Geometry check sheet. Reference: drawing and pictorial views, mm from the part's lowest x, y, z. Coordinates: 2 decimals unless noted, no trailing zeros. Loops run counter-clockwise (first coordinate to the right, second up) from the corner with the lowest first, then second, coordinate; pieces in that order, holes last.
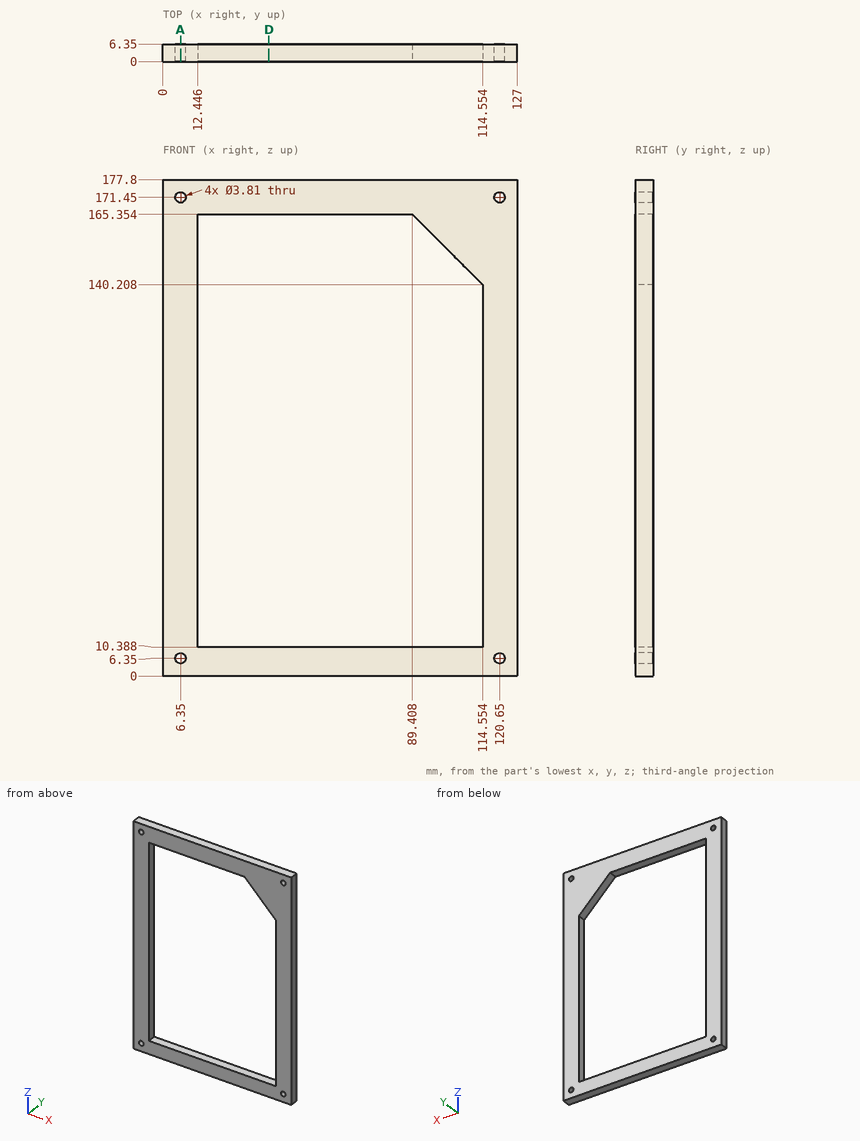
1) Section check D-D on x = 38. Record the cut outline in (y, z), and give its area (3 significant figures).
Data:
outline: (0, 0) - (6.35, 0) - (6.35, 10.39) - (0, 10.39) - close; (0, 165.35) - (6.35, 165.35) - (6.35, 177.8) - (0, 177.8) - close
area: 145 mm2
2) Material ranges on probe 1 along X at (y, z) = (4.5, 6.35) (1 decimal); probe 2 along Z at (x, y) = (64, 3.75); probe 3 along X at (y, z) = (3.5, 47), recorded low to high.
Data:
probe 1: x = 0 to 4.4, 8.3 to 118.7, 122.6 to 127
probe 2: z = 0 to 10.39, 165.35 to 177.8
probe 3: x = 0 to 12.45, 114.55 to 127
3) Section check A-A on x = 6.35. Count the separate pieces of the cut face and the enclosed holes in it, and give its area (3 significant figures).
Data:
separate pieces: 3
enclosed holes: 0
area: 1,080 mm2
4) Depth check by flat-ended pin: pin 1 (3 mm diameter, centred on x = 45.5, y = 4.5, fed in from -Z). Enter the tip coordinate at first touch or a pass-through.
Data:
pin 1: stops at z = 0
